from build123d import *

# Parameters (mm, degrees)
SKETCH1_W              = 70
SKETCH1_H              = 50
BOSS_EXTRUDE1_DEPTH    = 3
SKETCH2_W              = 3.5
SKETCH2_H              = 1.5
SKETCH2_W_2            = 1.5
SKETCH2_H_2            = 3.5
BOSS_EXTRUDE2_DEPTH    = 2.5
BOSS_EXTRUDE3_DEPTH    = 3
FILLET1_R              = 1
LPATTERN1_COUNT        = 2
LPATTERN1_PITCH        = 11.5
FILLET1_OF_LPATTERN1_R = 1
SKETCH6_R              = 1.5
BOSS_EXTRUDE4_DEPTH    = 2.5


with BuildPart() as part:
    # Sketch1 → Boss-Extrude1 (new body)
    with BuildSketch(Plane(origin=(0, 0, 0), x_dir=(1, 0, 0), z_dir=(0, 1, 0))):
        Rectangle(SKETCH1_W, SKETCH1_H)
    extrude(amount=BOSS_EXTRUDE1_DEPTH)

    # Sketch2 → Boss-Extrude2 (add)
    with BuildSketch(Plane.XZ):
        with Locations((0, 23.5)):
            Rectangle(SKETCH2_W, SKETCH2_H)
        with Locations((33.5, 0)):
            Rectangle(SKETCH2_W_2, SKETCH2_H_2)
        with Locations((-33.5, 0)):
            Rectangle(SKETCH2_W_2, SKETCH2_H_2)
    extrude(amount=BOSS_EXTRUDE2_DEPTH)

    # Sketch5 → Boss-Extrude3 (add)
    with BuildSketch(Plane.XY.offset(-15)):
        Polygon((35, 3), (35, 0), (45, 0), (45, 10), (-45, 10), (-45, 0), (-35, 0), (-35, 3), align=None)
    boss_extrude3 = extrude(amount=-BOSS_EXTRUDE3_DEPTH)

    # Fillet1
    fillet1_edges = [part.edges().sort_by_distance(p)[0] for p in [
        (-45, 0, -16.5),
        (-45, 10, -16.5),
        (45, 10, -16.5),
        (45, 0, -16.5),
    ]]
    fillet(fillet1_edges, radius=FILLET1_R)

    # LPattern1: Boss-Extrude3 ×2
    with Locations(*[(0, 0, i * LPATTERN1_PITCH) for i in range(1, LPATTERN1_COUNT)]):
        add(boss_extrude3)

    # Fillet1 of LPattern1
    fillet1_of_lpattern1_edges = [part.edges().sort_by_distance(p)[0] for p in [
        (-45, 0, -5),
        (-45, 10, -5),
        (45, 10, -5),
        (45, 0, -5),
    ]]
    fillet(fillet1_of_lpattern1_edges, radius=FILLET1_OF_LPATTERN1_R)

    # Sketch6 → Boss-Extrude4 (add, symmetric)
    with BuildSketch(Plane.ZY):
        with BuildLine():
            Line((-12.75, 0), (-8.75, 0))
            Line((-8.75, 0), (-8.75, 9))
            ThreePointArc((-8.75, 9), (-10.75, 11), (-12.75, 9))
            Line((-12.75, 9), (-12.75, 0))
        make_face()
        with Locations((-10.75, 9)):
            Circle(SKETCH6_R, mode=Mode.SUBTRACT)
    extrude(amount=BOSS_EXTRUDE4_DEPTH, both=True)


solid = part.part
Check sheet for the modelled part. Datum: model origin and axes. Units: mm. A direction names the side the tool comes from. Round coordinates to 2 decimals unless told otherwise and drop trailing zeros. Order: outer loops, then holes, each group sorted by start corner. A loop starts at its lowest first (then second) coordinate and runs counter-clockwise, first axis right, second up.
Q1. Depth check by flat-ended pin: P1, Ø1.2, axis at x = -33.5, y = -1.5, coming from the -Z side; P2, Ø5, axis at x = -7.5, z = 0, coming from the +Y side; P3, Ø2, axis at x = -20, z = -3.5, coming from the +Y side. Enter the tip coordinate at first touch or a pass-through.
Filled sheet:
P1: stops at z = -1.75
P2: stops at y = 3
P3: stops at y = 10
Q2. Cross-section at B-B, the plane y = 6.5. Enter the section's corners in (x, z).
Filled sheet:
outline: (-45, -18) - (45, -18) - (45, -15) - (-45, -15) - close; (-45, -6.5) - (45, -6.5) - (45, -3.5) - (-45, -3.5) - close; (-2.5, -12.75) - (2.5, -12.75) - (2.5, -8.75) - (-2.5, -8.75) - close
Q3. Set-up check for faces 4 (the face through (35, 1, -21)), 5 (the face through (35, 1, 11)), 6 (the face through (-35, 1, -21)), 7 (the face through (0, -1, 22.75)): record each of +Z, -Z, +X, -X, +Y, -Y from which the full face is reachable in a straight line by a thin tool's end or side.
Filled sheet:
face 4: -Z, +X, +Y, -Y
face 5: +Z, +X, +Y, -Y
face 6: -Z, -X, +Y, -Y
face 7: -Z, +X, -X, -Y
Q4. Cross-section at A-A, the plane z = -10.75. Enter the section's corners in (x, y), plus the area to 3 significant figures.
Filled sheet:
outline: (-35, 0) - (35, 0) - (35, 3) - (2.5, 3) - (2.5, 7.5) - (-2.5, 7.5) - (-2.5, 3) - (-35, 3) - close; (-2.5, 10.5) - (2.5, 10.5) - (2.5, 11) - (-2.5, 11) - close
area: 235 mm2
Q5. Draft check along X on faces 1 (the face through (32.75, -1, 0)), 2 (the face through (45, 5, -5)), 3 (the face through (0, 3, -22)). Enter one of: pulls with the +X half, pulls with the -X half, needs draft (parallel to the pull), parting line crosses it, or undercut.
Filled sheet:
face 1: undercut
face 2: pulls with the +X half
face 3: needs draft
Q6. Scan lines: L1, parallel to Z at x = 9.5, y = 8.75; L2, parallel to Y at x = -0.9, z = -10.75; L3, parallel to Y at x = -14, z = 22.5. Record each from-to range of solid material in increasing order.
Filled sheet:
L1: z = -18 to -15, -6.5 to -3.5
L2: y = 0 to 7.5, 10.5 to 11
L3: y = 0 to 3
Q7. Cross-section at C-C, the plane x = 19.5. Enter the section's corners in (y, z).
Filled sheet:
outline: (0, -25) - (3, -25) - (3, -18) - (10, -18) - (10, -15) - (3, -15) - (3, -6.5) - (10, -6.5) - (10, -3.5) - (3, -3.5) - (3, 25) - (0, 25) - close
